The listing builds one solid part. Answer for the finished solid, in the listing's coordinates (mm). Give positions to 0.01 mm unless a question says otherwise; leave off trailing zeros. Write each loop counter-clockwise with the first axis right and the second up, starting at its lowest first coordinate (ties: lowest second). Pieces come first, ordered by that corner, then holes.
Autodesk Inventor part; units mm, degrees
ref_plane "YZ Plane" through (0, 0, 0) normal (1, 0, 0) x (0, 1, 0)
ref_plane "XZ Plane" through (0, 0, 0) normal (0, 1, 0) x (-1, 0, 0)
ref_plane "XY Plane" through (0, 0, 0) normal (0, 0, 1) x (1, 0, 0)
sketch "Sketch9" plane through (0, 0, 0) normal (0, 1, 0) x (-1, 0, 0)
  arc A0 (-15.5418, 19.582) -> (-15.5418, -19.582) centre (0, 0) ccw
  arc A1 (-9.1876, -23.2506) -> (24.7294, -3.6686) centre (0, 0) ccw
  arc A2 (24.7294, 3.6686) -> (-9.1876, 23.2506) centre (0, 0) ccw
  circle A3 centre (0, 0) radius 25
  point P0 (-15.5418, -19.582)
  point P1 (-9.1876, -23.2506)
  point P2 (24.7294, -3.6686)
  point P3 (24.7294, 3.6686)
  point P4 (-15.5418, 19.582)
  dimension "d222" = 25
  dimension "d223" = 25
  dimension "d224" = 25
extrude "Extrusion4" add sketch "Sketch9" along normal blind 5
sketch "Sketch17" plane through (0, 5, 0) normal (0, 1, 0) x (1, 0, 0)
  arc A0 (15.5418, -19.582) -> (15.5418, 19.582) centre (0, 0) ccw
  line L0 (15.5418, 19.582) -> (24.6527, -4.1527)
  arc A1 (24.6527, -4.1527) -> (15.5418, 19.582) centre (0, 0) ccw
  line L1 (39.1744, 0) -> (-46.6954, 0) construction
  dimension "d244" = 69
extrude "Extrusion8" cut sketch "Sketch17" against normal through all
sketch "Sketch38" plane through (0, 5, 0) normal (0, 1, 0) x (1, 0, 0)
  line L0 (2.4652, 31.2084) -> (-0.476, 31.9965)
  line L1 (-0.476, 31.9965) -> (-11.5905, 25.0753)
  line L2 (8.3534, 21.0097) -> (2.4652, 31.2084)
  line L3 (-0.476, 31.9965) -> (2.4652, 31.2084)
  circle A0 centre (0, 0) radius 25
  line L4 (2.4652, 31.2084) -> (6.5546, 24.1255)
  arc A1 (6.2227, 24.2132) -> (14.6024, -20.2921) centre (0, 0) ccw
  line L5 (-11.0461, 17.1324) -> (-13.356, 21.1333)
  line L6 (-13.356, 21.1333) -> (-14.6216, 23.3253)
  line L7 (-14.6216, 23.3253) -> (-11.5905, 25.0753)
  line L8 (-13.356, 21.1333) -> (-6.4888, 10.7302)
  line L9 (-6.4888, 10.7302) -> (6.2227, 24.2132)
  point P0 (3.9242, 24.6901)
  point P1 (-24.7294, 3.6686)
  point P2 (9.1876, 23.2506)
  point P3 (8.9539, -17.5087)
  point P4 (6.5546, 24.1255)
extrude "Extrusion24" add sketch "Sketch38" against normal blind 5 contours L2 A0 L6 L7 L1 L0
sketch "Sketch43" plane through (0, 5, 0) normal (0, 1, 0) x (1, 0, 0)
  circle A0 centre (19.2133, -9.2784) radius 10
  arc A1 (12.0096, -16.2143) -> (26.417, -2.3425) centre (19.2133, -9.2784) ccw
  point P0 (0, 0)
  dimension "d385" = 20
extrude "Extrusion28" add sketch "Sketch43" against normal blind 5
properties part number "Electronic base"
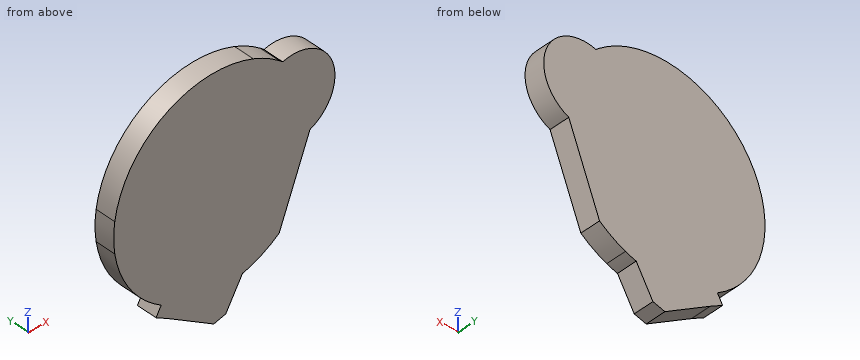
Item 1: A cutting plane is placed at B-B, the plane x = 13. Give the vertices of the cut face in (y, z).
Conclusion:
outline: (0, -21.35) - (5, -21.35) - (5, 21.35) - (0, 21.35) - close
Item 2: Consider probe 1 along X at (y, z) = (4.6, 6); probe 2 along X at (y, z) = (2.85, 17); probe 3 along Z at (x, y) = (0, 3.3). Determine where each line is inside the solid, lowest interval first.
Conclusion:
probe 1: x = -24.27 to 28.66
probe 2: x = -18.33 to 25.57
probe 3: z = -31.87 to 25
Item 3: A cutting plane is placed at A-A, the plane y = 3.2. Give the vertices of the cut face in (x, z), plus the area to 3 significant figures.
Conclusion:
outline: (-24.73, -3.67) arc R25 ccw to (-13.36, -21.13) - (-14.62, -23.33) - (-11.59, -25.08) - (-0.48, -32) - (2.47, -31.21) - (6.55, -24.13) arc R25 ccw to (9.19, -23.25) arc R25 ccw to (15.54, -19.58) - (23.08, 0.06) arc R10 ccw to (16.4, 18.87) arc R25 ccw to (15.54, 19.58) arc R25 ccw to (9.19, 23.25) arc R25 ccw to (-24.73, 3.67) arc R25 ccw to start
area: 2,090 mm2
Item 4: A cutting plane is placed at C-C, the plane z = -18.5. Give the vertices of the cut face in (x, y), plus the area to 3 significant figures.
Conclusion:
outline: (-16.82, 0) - (15.96, 0) - (15.96, 5) - (-16.82, 5) - close
area: 164 mm2
Item 5: Each of these flat-tipped pins is pushed along its axis until it touches: P1, Ø2, axis at x = -17.5, y = 4.5, coming from the +Z side; P2, Ø2, axis at y = 1.5, z = 3, coming from the +X side. Where does it stop, or does it pass through?
Conclusion:
P1: stops at z = 18.78
P2: stops at x = 27.71
